Here's the drawing with two shaded views (mm, measured from the low corner). I have some questions. A direction names the side the tool comes from. Round coordinates to 2 decimals unless told otherwise and drop trailing zeros. Loops run counter-clockwise (first coordinate to the right, second up) from the corner with the lowest first, then second, coordinate; pieces in that order, holes last.
(1) Which directions (+Z, -Z, +X, -X, +Y, -Y) give clear straight access to the entire face, cutting with the end or side of a thin tool? Please do the marked faces 1, 2 and 3.
(2) I want a section at C-C on z = 4.65. Write out the boundary of the cut face in (x, y).
(3) I want a section at D-D on y = 9.25. Write out the boundary of the cut face in (x, z), plus the area to 3 significant figures.
(4) If I drill on line 1 along Y through (x, z) = (10, 4.2); line 2 along X through (y, z) = (16.25, 3.9); line 3 along Z through (x, y) = (9.25, 6.75), over which ranges is the centre line in solid material (lowest first)?
(5) Will these pins go through, and if not, where does the flat tip stop? pin 1 Ø1 at (x, y) = (15, 22) entering from -Z; pin 2 Ø5.5 at (x, y) = (10, 16.5) entering from +Z; pin 3 Ø1.5 at (y, z) = (19.5, 1.5) entering from +X.
(6) Thinking about a two-plate mould opening in Y: for the marked faces 4, 5 and 6, which applies, released by +Y, released by -Y, zero draft, split by the parting line, or undercut?
(7) I want a section at B-B on y = 14. Write out the boundary of the cut face in (x, z).
(8) I want a section at A-A on x = 10. Write out the boundary of the cut face in (y, z).
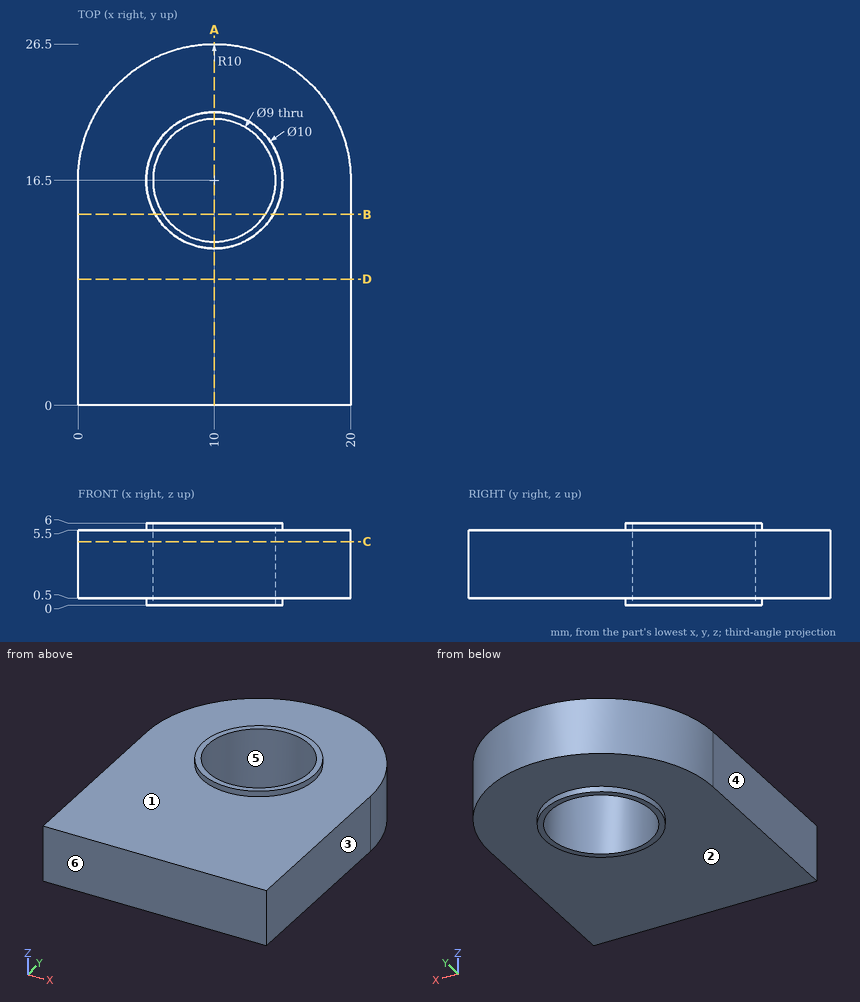
Filled sheet:
1. face 1: +Z
1. face 2: -Z
1. face 3: +Z, -Z, +X, +Y, -Y
2. outline: (0, 0) - (20, 0) - (20, 16.5) arc R10 ccw to (0, 16.5) - close; hole circle Ø9 at (10, 16.5)
3. outline: (0, 0.5) - (20, 0.5) - (20, 5.5) - (0, 5.5) - close
3. area: 100 mm2
4. line 1: y = 0 to 12, 21 to 26.5
4. line 2: x = 0 to 5.51, 14.49 to 20
4. line 3: z = 0.5 to 5.5
5. pin 1: stops at z = 0.5
5. pin 2: passes through
5. pin 3: stops at x = 19.74
6. face 4: zero draft
6. face 5: undercut
6. face 6: released by -Y
7. outline: (0, 0.5) - (5.67, 0.5) - (5.67, 0) - (6.26, 0) - (6.26, 6) - (5.67, 6) - (5.67, 5.5) - (0, 5.5) - close; (13.74, 0) - (14.33, 0) - (14.33, 0.5) - (20, 0.5) - (20, 5.5) - (14.33, 5.5) - (14.33, 6) - (13.74, 6) - close
8. outline: (0, 0.5) - (11.5, 0.5) - (11.5, 0) - (12, 0) - (12, 6) - (11.5, 6) - (11.5, 5.5) - (0, 5.5) - close; (21, 0) - (21.5, 0) - (21.5, 0.5) - (26.5, 0.5) - (26.5, 5.5) - (21.5, 5.5) - (21.5, 6) - (21, 6) - close
